Could you check a few things on this model? Use its own coordinates, in mm. A direction names the side the tool comes from. Round coordinates to 2 decimals unless told otherwise and drop trailing zeros. Write each loop counter-clockwise with the first axis right and the second up, starting at its lowest first coordinate (ties: lowest second). Pieces come first, ordered by that corner, then holes. Notation, with made-up numbers: M 86,-14 L 125,-14 A21 cw 125,-8 Z; hole C -12.75,-25.5 d1. An arc over 180 degrees is marked long. One line per item, written item: value. Start each with the question number.
(1) I want a section at B-B on z = 0. Please give me the cut outline in (x, y).
(2) I want a section at D-D on z = -10. Count the separate pieces of the cut face and the enclosed holes in it, and give its area (3 significant figures).
(3) I'm going to push flat-ended pins straight in: pin 1 Ø6 at (x, y) = (16.5, 2.5) entering from +Z; pin 2 Ø2 at (x, z) = (8, -21) entering from -Y; pin 3 Ø1.5 at (y, z) = (4, -11.5) entering from -X; pin 4 Ø11.5 at (x, z) = (-9, 6.5) entering from +Y. Where does each tip first touch, or does it pass through?
(4) If I drill on L1, parallel to X at y = 9.85, z = 0; L2, parallel to Z at x = -0.5, y = 8.5; L3, parallel to Y at x = 4, z = -10.5, over which ranges is the centre line in solid material (lowest first)?
(5) I want a section at C-C on y = 2. Please give me the cut outline in (x, z).
(6) Which directions (+Z, -Z, +X, -X, +Y, -Y) give clear straight access to the entire face, cutting with the end or side of a thin tool? Please do faces 1 (the face through (-17, 15, 18)), 2 (the face through (0, 4, 0)).
(7) I want a section at A-A on y = 7.75. Please give me the cut outline in (x, z), and give its area (3 significant figures).
(8) Thinking about a two-plate mould opening in X: for faces 3 (the face through (0, 0, 0)), 4 (the face through (-7.95, 2.03, -11.25)), 5 (the face through (-26.36, 7.93, -5.85)), which applies, released by +X, released by -X, zero draft, split by the parting line, or undercut?
```python
from build123d import *

# Parameters (mm, degrees)
SKETCH1_R           = 27
BOSS_EXTRUDE1_DEPTH = 15
SKETCH2_R           = 22.5
CUT_EXTRUDE1_DEPTH  = 11
FILLET1_R           = 3
FILLET2_R           = 3
FILLET3_R           = 2
FILLET4_R           = 2
SKETCH4_R           = 1.25
CUT_EXTRUDE2_DEPTH  = 11


with BuildPart() as part:
    # Sketch1 → Boss-Extrude1 (new body)
    with BuildSketch(Plane(origin=(0, 0, 0), x_dir=(1, 0, 0), z_dir=(0, 1, 0))):
        with Locations(Location((0, 0, 0), (0, 0, 270))):
            Circle(SKETCH1_R)
    extrude(amount=BOSS_EXTRUDE1_DEPTH)

    # Sketch2 → Cut-Extrude1 (cut)
    with BuildSketch(Plane(origin=(0, 15, 0), x_dir=(1, 0, 0), z_dir=(0, 1, 0))):
        with Locations(Location((0, 0, 0), (0, 0, 270))):
            Circle(SKETCH2_R)
    extrude(amount=-CUT_EXTRUDE1_DEPTH, mode=Mode.SUBTRACT)

    # Fillet1
    fillet1_edges = [part.edges().sort_by_distance(p)[0] for p in [
        (0, 0, -27),
    ]]
    fillet(fillet1_edges, radius=FILLET1_R)

    # Fillet2
    fillet2_edges = [part.edges().sort_by_distance(p)[0] for p in [
        (0, 4, -22.5),
    ]]
    fillet(fillet2_edges, radius=FILLET2_R)

    # Fillet3
    fillet3_edges = [part.edges().sort_by_distance(p)[0] for p in [
        (0, 15, -27),
    ]]
    fillet(fillet3_edges, radius=FILLET3_R)

    # Fillet4
    fillet4_edges = [part.edges().sort_by_distance(p)[0] for p in [
        (0, 15, -22.5),
    ]]
    fillet(fillet4_edges, radius=FILLET4_R)

    # Sketch4 → Cut-Extrude2 (cut)
    with BuildSketch(Plane(origin=(0, 4, 0), x_dir=(1, 0, 0), z_dir=(0, 1, 0))):
        with Locations(Location((-8, 10, 0), (0, 0, 270))):
            Circle(SKETCH4_R)
        with Locations(Location((8, 10, 0), (0, 0, 270))):
            Circle(SKETCH4_R)
        with Locations(Location((0, 15, 0), (0, 0, 270))):
            Circle(SKETCH4_R)
    extrude(amount=-CUT_EXTRUDE2_DEPTH, mode=Mode.SUBTRACT)


solid = part.part
```
Found:
1. outline: M -27,3 A3 ccw -24,0 L 24,0 A3 ccw 27,3 L 27,13 A2 ccw 25,15 L 24.5,15 A2 ccw 22.5,13 L 22.5,7 A3 cw 19.5,4 L -19.5,4 A3 cw -22.5,7 L -22.5,13 A2 ccw -24.5,15 L -25,15 A2 ccw -27,13 Z
2. separate pieces: 3
2. enclosed holes: 0
2. area: 285 mm²
3. pin 1: stops at z = 23.37
3. pin 2: stops at y = 0
3. pin 3: stops at x = -24.77
3. pin 4: stops at y = 4
4. L1: x = -27 to -22.5, 22.5 to 27
4. L2: z = -27 to -22.49, 22.49 to 27
4. L3: y = 0 to 4
5. outline: C 0,0 d53.66; hole C -8,-10 d2.5; hole C 0,-15 d2.5; hole C 8,-10 d2.5
6. face 1: +Z, -Z, +X, -X, +Y
6. face 2: +Y
7. outline: C 0,0 d54; hole C 0,0 d45
7. area: 700 mm²
8. face 3: zero draft
8. face 4: undercut
8. face 5: split by the parting line
